Source: CAD feature listing. Evaluate the final solid. Frame: model axes, mm. A direction names the side the tool comes from. Give positions to 0.01 mm unless a question says otherwise; leave off trailing zeros. Order: outer loops, then holes, each group sorted by start corner. A loop starts at its lowest first (then second) coordinate and runs counter-clockwise, first axis right, second up.
1) Access query for faces 4 (the face through (-36.27, 37.75, 5.68)), 5 (the face through (0, 34, 1.2)). Directions: +Z, -Z, +X, -X, +Y, -Y. A direction counts if a zero-diameter tool reaches every point of the face in a straight line with its end or side. Return the directions, or none.
2) First-contact query: P1, Ø3, axis at x = -34, y = -34, coming from the -Z side; P2, Ø0.7, axis at x = -0.5, y = 34, coming from the +Z side. Flat tips, straight axial feed; report the tip coordinate or a pass-through.
3) Section B-B, the plane x = 0. Return loops of the section in (y, z), plus the area to 3 significant figures.
4) Section C-C, the plane x = -21.5. Return loops of the section in (y, z), plus the area to 3 significant figures.
5) Section A-A, the plane z = 7.75. Return loops of the section in (x, y).
6) Material intervals for line 1 (Y direction, x = 0, z = 4.75); line 2 (X direction, y = -34, z = 8.25); line 3 (X direction, y = 18, z = 8.25), sorted ascending.
7) Draft query along X for faces 1 (the face through (-37.7, 0, 6)), 2 (the face through (0, 29, 11.2)), 3 (the face through (0, -34, 1.2)). Return one class per face: released by +X, released by -X, zero draft, split by the parting line, or undercut.
```python
from build123d import *

# Parameters (mm, degrees)
SKETCH1_W                                         = 75.4
SKETCH1_H                                         = 78.5
BOSS_EXTRUDE1_DEPTH                               = 11.2
SKETCH2_W                                         = 69
SKETCH2_H                                         = 49
CUT_EXTRUDE1_DEPTH                                = 10
FILLET2_R                                         = 2
SKETCH3_R                                         = 1.2446
CUT_EXTRUDE2_DEPTH                                = 10
FILLET3_R                                         = 5
CSK_FOR_4_FLAT_HEAD_MACHINE_SCREW_100_D           = 3.4544
CSK_FOR_4_FLAT_HEAD_MACHINE_SCREW_100_CSINK_D     = 5.715
CSK_FOR_4_FLAT_HEAD_MACHINE_SCREW_100_CSINK_ANGLE = 100


with BuildPart() as part:
    # Sketch1 → Boss-Extrude1 (new body)
    with BuildSketch(Plane.XY):
        Rectangle(SKETCH1_W, SKETCH1_H)
    extrude(amount=BOSS_EXTRUDE1_DEPTH)

    # Sketch2 → Cut-Extrude1 (cut)
    with BuildSketch(Plane.XY.offset(11.2)):
        Rectangle(SKETCH2_W, SKETCH2_H)
    extrude(amount=-CUT_EXTRUDE1_DEPTH, mode=Mode.SUBTRACT)

    # Fillet2
    fillet2_edges = [part.edges().sort_by_distance(p)[0] for p in [
        (34.5, 0, 11.2),
        (0, 24.5, 11.2),
        (-34.5, 0, 11.2),
        (0, -24.5, 11.2),
    ]]
    fillet(fillet2_edges, radius=FILLET2_R)

    # Sketch3 → Cut-Extrude2 (cut)
    with BuildSketch(Plane.XY.offset(11.2)):
        with Locations((0, 34)):
            Circle(SKETCH3_R)
        with Locations(Location((0, -34, 0), (0, 0, 180))):
            Circle(SKETCH3_R)
    extrude(amount=-CUT_EXTRUDE2_DEPTH, mode=Mode.SUBTRACT)

    # Fillet3
    fillet3_edges = [part.edges().sort_by_distance(p)[0] for p in [
        (37.7, -39.25, 5.6),
        (-37.7, -39.25, 5.6),
        (-37.7, 39.25, 5.6),
        (37.7, 39.25, 5.6),
    ]]
    fillet(fillet3_edges, radius=FILLET3_R)

    # CSK for #4 Flat Head Machine Screw (100)1 (through all)
    with Locations(Plane.XY.offset(11.2)):
        with Locations((34, -34), (-34, -34), (-34, 34), (34, 34)):
            CounterSinkHole(CSK_FOR_4_FLAT_HEAD_MACHINE_SCREW_100_D / 2, CSK_FOR_4_FLAT_HEAD_MACHINE_SCREW_100_CSINK_D / 2, counter_sink_angle=CSK_FOR_4_FLAT_HEAD_MACHINE_SCREW_100_CSINK_ANGLE)


solid = part.part
```
From the geometry:
1. face 4: +Z, -Z, -X, +Y
1. face 5: +Z
2. P1: passes through
2. P2: stops at z = 1.2
3. outline: (-39.25, 0) - (39.25, 0) - (39.25, 11.2) - (35.24, 11.2) - (35.24, 1.2) - (32.76, 1.2) - (32.76, 11.2) - (26.5, 11.2) arc R2 ccw to (24.5, 9.2) - (24.5, 1.2) - (-24.5, 1.2) - (-24.5, 9.2) arc R2 ccw to (-26.5, 11.2) - (-32.76, 11.2) - (-32.76, 1.2) - (-35.24, 1.2) - (-35.24, 11.2) - (-39.25, 11.2) - close
3. area: 338 mm2
4. outline: (-39.25, 0) - (39.25, 0) - (39.25, 11.2) - (26.5, 11.2) arc R2 ccw to (24.5, 9.2) - (24.5, 1.2) - (-24.5, 1.2) - (-24.5, 9.2) arc R2 ccw to (-26.5, 11.2) - (-39.25, 11.2) - close
4. area: 387 mm2
5. outline: (-37.7, -34.25) arc R5 ccw to (-32.7, -39.25) - (32.7, -39.25) arc R5 ccw to (37.7, -34.25) - (37.7, 34.25) arc R5 ccw to (32.7, 39.25) - (-32.7, 39.25) arc R5 ccw to (-37.7, 34.25) - close; hole circle Ø3.45 at (-34, -34); hole circle Ø3.45 at (-34, 34); hole (-34.5, -24.5) - (34.5, -24.5) - (34.5, 24.5) - (-34.5, 24.5) - close; hole circle Ø2.49 at (0, -34); hole circle Ø2.49 at (0, 34); hole circle Ø3.45 at (34, -34); hole circle Ø3.45 at (34, 34)
6. line 1: y = -39.25 to -35.24, -32.76 to -24.5, 24.5 to 32.76, 35.24 to 39.25
6. line 2: x = -37.7 to -35.73, -32.27 to -1.24, 1.24 to 32.27, 35.73 to 37.7
6. line 3: x = -37.7 to -34.5, 34.5 to 37.7
7. face 1: released by -X
7. face 2: zero draft
7. face 3: undercut
